Geometry: final body of the model. Coordinates: model frame, mm. A direction names the side the tool comes from. Coordinates: 2 decimals unless noted, no trailing zeros. Loops run counter-clockwise (first coordinate to the right, second up) from the corner with the lowest first, then second, coordinate; pieces in that order, holes last. Notation, with made-up numbers: (84, -16) - (103, -16) arc R27 cw to (103, 5) - close; hole circle Ø3 at (27.5, 49.25). An arc over 180 degrees is marked (long way). Answer in a Markdown table with one row per item.
from build123d import *

# Parameters (mm, degrees)
ESQUISSE4_R                   = 13.9
ESQUISSE4_R_2                 = 1.55
BOSS_EXTRU_3_DEPTH            = 4.5
ESQUISSE7_R                   = 15.9
ESQUISSE7_R_2                 = 13.9
BOSS_EXTRU_7_DEPTH            = 9
BOSS_EXTRU_8_DEPTH            = 30
ENL_V_START                   = -4.5
ENL_V_MAT_EXTRU_12_OUTLINE_R  = 1.55
ENL_V_MAT_EXTRU_12_DEPTH      = 9
TROU_TARAUD_M32_D             = 2.5
TROU_TARAUD_M32_DEPTH         = 26.66
TROU_TARAUD_M32_CSINK_D       = 3.5
TROU_TARAUD_M32_CSINK_ANGLE   = 90
ENL_V_MAT_EXTRU_1_DEPTH       = 22
ESQUISSE13_R                  = 2.05
ENL_V_MAT_EXTRU_4_DEPTH       = 65.256925163
ESQUISSE15_R                  = 2.05
ENL_V_MAT_EXTRU_5_DEPTH       = 61.387436039
ENL_V_MAT_EXTRU_6_DEPTH       = 73.985973625
ESQUISSE24_R                  = 4.05
ENL_V_MAT_EXTRU_9_DEPTH       = 2.5
TROU_TARAUD_M33_D             = 2.5
TROU_TARAUD_M33_DEPTH         = 23.155777755
TROU_TARAUD_M33_CSINK_D       = 3.5
TROU_TARAUD_M33_CSINK_ANGLE   = 90
CONG_2_R                      = 1
ENL_V_MAT_EXTRU_13_DEPTH      = 57.002436454
ENL_V_MAT_EXTRU_13_DEPTH_BACK = 57.002436454
CONG_3_R                      = 1
CONG_4_R                      = 1


# Read off the part's stored shape, not the designer's step: Enlèv. mat.-Extru.12
with BuildPart() as part:
    # Esquisse4 → Boss.-Extru.3 (new, symmetric)
    with BuildSketch(Plane.XY):
        Circle(ESQUISSE4_R)
        with Locations((-6.717514421, -6.717514421)):
            Circle(ESQUISSE4_R_2, mode=Mode.SUBTRACT)
        with Locations((6.717514421, 6.717514421)):
            Circle(ESQUISSE4_R_2, mode=Mode.SUBTRACT)
        with Locations((-5.656854249, 5.656854249)):
            Circle(ESQUISSE4_R_2, mode=Mode.SUBTRACT)
        with Locations((5.656854249, -5.656854249)):
            Circle(ESQUISSE4_R_2, mode=Mode.SUBTRACT)
        with BuildLine():
            ThreePointArc((-10.594734512, 6.911881121), (-12.65, 0), (-10.594734512, -6.911881121))
            ThreePointArc((-10.594734512, -6.911881121), (-7.999175124, 0), (-10.594734512, 6.911881121))
        make_face(mode=Mode.SUBTRACT)
        with BuildLine():
            ThreePointArc((6.911881121, -10.594734512), (0, -7.999175124), (-6.911881121, -10.594734512))
            ThreePointArc((-6.911881121, -10.594734512), (0, -12.65), (6.911881121, -10.594734512))
        make_face(mode=Mode.SUBTRACT)
        with BuildLine():
            ThreePointArc((-6.911881121, 10.594734512), (0, 7.999175124), (6.911881121, 10.594734512))
            ThreePointArc((6.911881121, 10.594734512), (0, 12.65), (-6.911881121, 10.594734512))
        make_face(mode=Mode.SUBTRACT)
        with BuildLine():
            ThreePointArc((10.594734512, 6.911881121), (7.999175124, 0), (10.594734512, -6.911881121))
            ThreePointArc((10.594734512, -6.911881121), (12.65, 0), (10.594734512, 6.911881121))
        make_face(mode=Mode.SUBTRACT)
    extrude(amount=BOSS_EXTRU_3_DEPTH, both=True)

    # Esquisse7 → Boss.-Extru.7 (add)
    with BuildSketch(Plane.XY.offset(4.5)):
        Circle(ESQUISSE7_R)
        Circle(ESQUISSE7_R_2, mode=Mode.SUBTRACT)
    extrude(amount=-BOSS_EXTRU_7_DEPTH)

    # Esquisse6 → Boss.-Extru.8 (add)
    with BuildSketch(Plane(origin=(0, -15, 0), x_dir=(1, 0, 0), z_dir=(0, 1, 0))):
        Polygon((-51.798424989, -22.16), (-29.798424989, -22.16), (-15.9, -4.5), (0, -4.5), (0, 4.5), (-15.9, 4.5), (-51.798424989, 4.5), align=None)
    extrude(amount=BOSS_EXTRU_8_DEPTH)

    # Enlèv. mat.-Extru.12 outline → Enlèv. mat.-Extru.12 (cut)
    with BuildSketch(Plane.XY.offset(ENL_V_START)):
        with BuildLine():
            ThreePointArc((0, 12.65), (-3.605489456, 12.125301884), (-6.911881121, 10.594734512))
            ThreePointArc((-6.911881121, 10.594734512), (-6.773099648, 10.475509721), (-6.632262004, 10.358720998))
            ThreePointArc((-6.632262004, 10.358720998), (-6.631896353, 10.3589551), (-6.631530694, 10.359189189))
            ThreePointArc((-6.631530694, 10.359189189), (-3.519338467, 8.607363508), (0, 8))
            Line((0, 8), (0, 12.65))
        make_face()
        with BuildLine():
            ThreePointArc((-6.911881121, -10.594734512), (-3.605489456, -12.125301884), (0, -12.65))
            Line((0, -12.65), (0, -8))
            ThreePointArc((0, -8), (-3.519338467, -8.607363508), (-6.631530694, -10.359189189))
            ThreePointArc((-6.631530694, -10.359189189), (-6.631896353, -10.3589551), (-6.632262004, -10.358720998))
            ThreePointArc((-6.632262004, -10.358720998), (-6.773099648, -10.475509721), (-6.911881121, -10.594734512))
        make_face()
        with BuildLine():
            ThreePointArc((-10.358720998, 6.632262004), (-10.475509721, 6.773099648), (-10.594734512, 6.911881121))
            ThreePointArc((-10.594734512, 6.911881121), (-12.65, 0), (-10.594734512, -6.911881121))
            ThreePointArc((-10.594734512, -6.911881121), (-10.475509721, -6.773099648), (-10.358720998, -6.632262004))
            ThreePointArc((-10.358720998, -6.632262004), (-10.3589551, -6.631896353), (-10.359189189, -6.631530694))
            ThreePointArc((-10.359189189, -6.631530694), (-8, 0), (-10.359189189, 6.631530694))
            ThreePointArc((-10.359189189, 6.631530694), (-10.3589551, 6.631896353), (-10.358720998, 6.632262004))
        make_face()
        with Locations((-6.717514421, -6.717514421)):
            Circle(ENL_V_MAT_EXTRU_12_OUTLINE_R)
        with Locations((-5.656854249, 5.656854249)):
            Circle(ENL_V_MAT_EXTRU_12_OUTLINE_R)
    extrude(amount=ENL_V_MAT_EXTRU_12_DEPTH, mode=Mode.SUBTRACT)

    # Trou taraudé M32
    with Locations(Plane(origin=(5.656854249, -5.656854249, -4.5), x_dir=(-1, 0, 0), z_dir=(0, 0, -1))):
        with Locations((0, 0), (-1.060660172, 12.37436867)):
            CounterSinkHole(TROU_TARAUD_M32_D / 2, TROU_TARAUD_M32_CSINK_D / 2, depth=TROU_TARAUD_M32_DEPTH, counter_sink_angle=TROU_TARAUD_M32_CSINK_ANGLE)

    # Esquisse8 → Enlèv. mat.-Extru.1 (cut)
    with BuildSketch(Plane.ZY.offset(51.798424989)):
        with BuildLine():
            Line((19, 10.05), (2, 10.05))
            ThreePointArc((2, 10.05), (0.939339828, 9.610660172), (0.5, 8.55))
            Line((0.5, 8.55), (0.5, -8.55))
            ThreePointArc((0.5, -8.55), (0.939339828, -9.610660172), (2, -10.05))
            Line((2, -10.05), (19, -10.05))
            ThreePointArc((19, -10.05), (20.060660172, -9.610660172), (20.5, -8.55))
            Line((20.5, -8.55), (20.5, 8.55))
            ThreePointArc((20.5, 8.55), (20.060660172, 9.610660172), (19, 10.05))
        make_face()
    extrude(amount=-ENL_V_MAT_EXTRU_1_DEPTH, mode=Mode.SUBTRACT)

    # Esquisse13 → Enlèv. mat.-Extru.4 (cut, through all)
    with BuildSketch(Plane.XZ.offset(15)):
        with Locations(Location((-40.798424989, 10.5, 0), (0, 0, 270))):
            Circle(ESQUISSE13_R)
    extrude(amount=-ENL_V_MAT_EXTRU_4_DEPTH, mode=Mode.SUBTRACT)

    # Esquisse15 → Enlèv. mat.-Extru.5 (cut, through all)
    with BuildSketch(Plane(origin=(0, 0, -4.5), x_dir=(-1, 0, 0), z_dir=(0, 0, -1))):
        with Locations((40.798424989, 0)):
            Circle(ESQUISSE15_R)
    extrude(amount=-ENL_V_MAT_EXTRU_5_DEPTH, mode=Mode.SUBTRACT)

    # Esquisse16 → Enlèv. mat.-Extru.6 (cut, through all)
    with BuildSketch(Plane.ZY.offset(51.798424989)):
        Polygon((18.655777755, 10.05), (18.655777755, -10.05), (18.655777755, -15), (22.16, -15), (22.16, 15), (18.655777755, 15), align=None)
    extrude(amount=-ENL_V_MAT_EXTRU_6_DEPTH, mode=Mode.SUBTRACT)

    # Esquisse24 → Enlèv. mat.-Extru.9 (cut)
    with BuildSketch(Plane.XY.offset(4.5)):
        Circle(ESQUISSE24_R)
    extrude(amount=-ENL_V_MAT_EXTRU_9_DEPTH, mode=Mode.SUBTRACT)

    # Trou taraudé M33
    with Locations(Plane(origin=(0, 0, -4.5), x_dir=(-1, 0, 0), z_dir=(0, 0, -1))):
        with Locations((6.717514421, -6.717514421), (5.656854249, 5.656854249)):
            CounterSinkHole(TROU_TARAUD_M33_D / 2, TROU_TARAUD_M33_CSINK_D / 2, depth=TROU_TARAUD_M33_DEPTH, counter_sink_angle=TROU_TARAUD_M33_CSINK_ANGLE)

    # Congé2
    cong_2_edges = [part.edges().sort_by_distance(p)[0] for p in [
        (-21.470300546, -15, 11.577888877),
        (-21.470300546, 15, 11.577888877),
        (-39.419513041, 15, 18.655777755),
        (-27.040601092, 0, 18.655777755),
        (-39.419513041, -15, 18.655777755),
        (15.9, 0, -4.5),
        (15.9, 0, 4.5),
        (-15.9, 0, 4.5),
        (-10.586759375, -15, 4.5),
        (-28.535971869, -15, -4.5),
        (-51.798424989, 0, -4.5),
        (-28.535971869, 15, -4.5),
        (-10.586759375, 15, 4.5),
    ]]
    fillet(cong_2_edges, radius=CONG_2_R)

    # Esquisse27 → Enlèv. mat.-Extru.13 (cut, two sides: drawn at the far end of the back side and taken through both)
    with BuildSketch(Plane.XY.offset(4.5).offset(-ENL_V_MAT_EXTRU_13_DEPTH_BACK)):
        with BuildLine():
            Line((-18.443262039, -10.5), (-21.520938865, -10.5))
            Line((-21.520938865, -10.5), (-21.520938865, 10.5))
            Line((-21.520938865, 10.5), (-18.443262039, 10.5))
            ThreePointArc((-18.443262039, 10.5), (-7.943262039, 0), (-18.443262039, -10.5))
        make_face()
    extrude(amount=ENL_V_MAT_EXTRU_13_DEPTH + ENL_V_MAT_EXTRU_13_DEPTH_BACK, mode=Mode.SUBTRACT)

    # Congé3
    cong_3_edges = [part.edges().sort_by_distance(p)[0] for p in [
        (-21.520938865, 10.5, 3.571116167),
        (-21.520938865, -10.5, 3.571116167),
    ]]
    fillet(cong_3_edges, radius=CONG_3_R)

    # Congé4
    # the kernel refuses this fillet: 1 mm, written as the material it takes off along each edge
    with BuildSketch(Plane(origin=(-50.798424989, 14, -3.5), x_dir=(-1, 0, 0), z_dir=(0, 1, 0))) as cong_4_piece_1_section:
        Polygon((0, 0), (CONG_4_R, 0), (CONG_4_R, -CONG_4_R), (0, -CONG_4_R), align=None)
    cong_4_piece_1 = extrude(amount=CONG_4_R, mode=Mode.PRIVATE)
    cong_4_piece_1 = cong_4_piece_1 - Plane(origin=(-50.798424989, 14, -3.5), x_dir=(0.7071067811865477, 0, 0.7071067811865475), z_dir=(0, 1, 0)) * Sphere(CONG_4_R, mode=Mode.PRIVATE)
    add(cong_4_piece_1, mode=Mode.SUBTRACT)
    with BuildSketch(Plane(origin=(-50.798424989, -14, -3.5), x_dir=(-1, 0, 0), z_dir=(0, -1, 0))) as cong_4_piece_2_section:
        Polygon((0, 0), (CONG_4_R, 0), (CONG_4_R, CONG_4_R), (0, CONG_4_R), align=None)
    cong_4_piece_2 = extrude(amount=CONG_4_R, mode=Mode.PRIVATE)
    cong_4_piece_2 = cong_4_piece_2 - Plane(origin=(-50.798424989, -14, -3.5), x_dir=(0.7071067811865477, 0, 0.7071067811865475), z_dir=(0, -1, 0)) * Sphere(CONG_4_R, mode=Mode.PRIVATE)
    add(cong_4_piece_2, mode=Mode.SUBTRACT)
    with BuildSketch(Plane(origin=(-51.798424989, -14, 18.655777755), x_dir=(1, 0, 0), z_dir=(0, 1, 0)), Plane(origin=(-51.798424989, 7.55, 18.655777755), x_dir=(1, 0, 0), z_dir=(0, 1, 0))) as cong_4_piece_3:
        with BuildLine():
            CenterArc((CONG_4_R, CONG_4_R), CONG_4_R, 180, 90)
            Line((0, CONG_4_R), (0, 0))
            Line((0, 0), (CONG_4_R, 0))
        make_face()
    extrude(amount=6.45, mode=Mode.SUBTRACT)
    with BuildSketch(Plane(origin=(-51.798424989, -15, -3.5), x_dir=(1, 0, 0), z_dir=(0, 0, 1))) as cong_4_piece_4:
        with BuildLine():
            CenterArc((CONG_4_R, CONG_4_R), CONG_4_R, 180, 90)
            Line((0, CONG_4_R), (0, 0))
            Line((0, 0), (CONG_4_R, 0))
        make_face()
    extrude(amount=21.155777755, mode=Mode.SUBTRACT)
    with BuildSketch(Plane(origin=(-51.798424989, 15, -3.5), x_dir=(1, 0, 0), z_dir=(0, 0, 1))) as cong_4_piece_5:
        with BuildLine():
            CenterArc((CONG_4_R, -CONG_4_R), CONG_4_R, 90, 90)
            Line((0, -CONG_4_R), (0, 0))
            Line((0, 0), (CONG_4_R, 0))
        make_face()
    extrude(amount=21.155777755, mode=Mode.SUBTRACT)
    with BuildSketch(Plane(origin=(-51.798424989, 14, 17.655777755), x_dir=(0, 0, 1), z_dir=(0, -1, 0))) as cong_4_piece_6:
        with BuildLine():
            CenterArc((1 - CONG_4_R, -CONG_4_R), CONG_4_R, 0, 90)
            Line((1, -CONG_4_R), (1, 0))
            Line((1, 0), (1 - CONG_4_R, 0))
        make_face()
    revolve(axis=Axis((-51.798424989, 14, 17.655777755), (-1, 0, 0)), revolution_arc=90, mode=Mode.SUBTRACT)
    with BuildSketch(Plane(origin=(-51.798424989, -14, 17.655777755), x_dir=(0, 0, 1), z_dir=(0, 1, 0))) as cong_4_piece_7:
        with BuildLine():
            CenterArc((1 - CONG_4_R, CONG_4_R), CONG_4_R, 270, 90)
            Line((1 - CONG_4_R, 0), (1, 0))
            Line((1, 0), (1, CONG_4_R))
        make_face()
    revolve(axis=Axis((-51.798424989, -14, 17.655777755), (1, 0, 0)), revolution_arc=90, mode=Mode.SUBTRACT)


solid = part.part
(1) Pull-direction query (Y, two-part tool) for faces 1 (the face through (15.894, -0.425, 0.049)), 2 (the face through (-51.798, 0, 0)), 3 (the face through (-3.5, -8.6, -0.1)); classes: pulls with the +Y half, pulls with the -Y half, needs draft (parallel to the pull), parting line crosses it, or undercut.
Verdict:
| item | result |
|---|---|
| face 1 | parting line crosses it |
| face 2 | needs draft |
| face 3 | undercut |
(2) First-contact query: pin 1 Ø2 at (x, y) = (-17.5, -10.5) entering from +Z; pin 2 Ø3 at (y, z) = (9, 11.5) entering from -X; pin 3 Ø2 at (x, y) = (4.5, -7.5) entering from +Z; pin 4 Ø13.5 at (x, z) = (-36.5, 8) entering from -Y. Flat tips, straight axial feed; report the tip coordinate or a pass-through.
Verdict:
| item | result |
|---|---|
| pin 1 | stops at z = 7.8 |
| pin 2 | stops at x = -51.8 |
| pin 3 | stops at z = 4.5 |
| pin 4 | stops at y = -15 |
(3) Ray query, probe 1 along Y at (x, z) = (1.5, 1.25); probe 2 along Y at (x, z) = (-26, 3.5); probe 3 along Y at (x, z) = (-43.5, 15). Return the intervals inside material, ascending.
Verdict:
| item | result |
|---|---|
| probe 1 | y = -15.83 to -12.56, -8.11 to 8.11, 12.56 to 15.83 |
| probe 2 | y = -15 to 15 |
| probe 3 | y = -15 to -10.05, 10.05 to 15 |
(4) Access query for faces 4 (the face through (-43, 10.05, 10)), 5 (the face through (0, 0, 2)), 6 (the face through (-33, -15, 5)), 7 (the face through (-39.4, 12.5, 12)), 8 (the face through (-7.946, 0.231, 0.171)). Directions: +Z, -Z, +X, -X, +Y, -Y. A direction counts if a zero-diameter tool reaches every point of the face in a straight line with its end or side. Return the directions, or none.
Verdict:
| item | result |
|---|---|
| face 4 | +Z, -X |
| face 5 | +Z |
| face 6 | +Z, -Z, -X, -Y |
| face 7 | +Y, -Y |
| face 8 | +Z, -Z |
(5) Cut plane D-D on x = -1. State how many separate pieces and enclosed holes the cut face has, then the cut area to 3 significant figures.
Verdict:
| item | result |
|---|---|
| separate pieces | 3 |
| enclosed holes | 0 |
| area | 183 mm² |
(6) Cut plane C-C on x = -39.5. Output: boundary loops of the cut face in (y, z), then the cut area to 3 significant figures.
Verdict:
| item | result |
|---|---|
| outline | (-15, -3.5) arc R1 ccw to (-14, -4.5) - (-1.59, -4.5) - (-1.59, 0.5) - (-8.55, 0.5) arc R1.5 cw to (-10.05, 2) - (-10.05, 8.91) - (-15, 8.91) - close; (-15, 12.09) - (-10.05, 12.09) - (-10.05, 18.66) - (-14, 18.66) arc R1 ccw to (-15, 17.66) - close; (1.59, -4.5) - (14, -4.5) arc R1 ccw to (15, -3.5) - (15, 8.91) - (10.05, 8.91) - (10.05, 2) arc R1.5 cw to (8.55, 0.5) - (1.59, 0.5) - close; (10.05, 12.09) - (15, 12.09) - (15, 17.66) arc R1 ccw to (14, 18.66) - (10.05, 18.66) - close |
| area | 283 mm² |
(7) Cut plane A-A on y = 0. Output: boundary loops of the cut face in (x, z), then the cut area to 3 significant figures.
Verdict:
| item | result |
|---|---|
| outline | (-51.8, -3.5) arc R1 ccw to (-50.8, -4.5) - (-42.85, -4.5) - (-42.85, 0.5) - (-51.8, 0.5) - close; (-38.75, -4.5) - (-21.52, -4.5) - (-21.52, 11.64) - (-26.74, 18.27) arc R1 ccw to (-27.53, 18.66) - (-29.8, 18.66) - (-29.8, 0.5) - (-38.75, 0.5) - close; (-7.94, -4.5) - (8, -4.5) - (8, 4.5) - (4.05, 4.5) - (4.05, 2) - (-4.05, 2) - (-4.05, 4.5) - (-7.94, 4.5) - close; (12.65, -4.5) - (14.9, -4.5) arc R1 ccw to (15.9, -3.5) - (15.9, 3.5) arc R1 ccw to (14.9, 4.5) - (12.65, 4.5) - close |
| area | 414 mm² |
(8) Cut plane B-B on x = -31.5. Output: boundary loops of the cut face in (y, z).
Verdict:
| item | result |
|---|---|
| outline | (-15, -3.5) arc R1 ccw to (-14, -4.5) - (14, -4.5) arc R1 ccw to (15, -3.5) - (15, 17.66) arc R1 ccw to (14, 18.66) - (10.05, 18.66) - (10.05, 2) arc R1.5 cw to (8.55, 0.5) - (-8.55, 0.5) arc R1.5 cw to (-10.05, 2) - (-10.05, 18.66) - (-14, 18.66) arc R1 ccw to (-15, 17.66) - close |
